Can you work these out from the model? Positions are in its coordinate system, mm. A direction names the side the tool comes from. Give positions to 0.01 mm unless a question says otherwise; leave off trailing zeros. Loops run counter-clockwise (first coordinate to the right, second up) from the corner with the lowest first, then second, coordinate; pieces in that order, holes last. Notation, with made-up numbers: (13, 37.5) - (46, 37.5) arc R17 cw to (46, 41.5) - close; hole circle Ø5 at (49, 89.25). An arc over 180 degrees is marked (long way). Answer as a JSON object with one key per item and string values.
```python
from build123d import *

# Parameters (mm, degrees)
ESBO_O1_W                = 60
ESBO_O1_H                = 50
RESSALTO_EXTRUS_O1_DEPTH = 50
ESBO_O2_W                = 60
ESBO_O2_H                = 29
CORTE_EXTRUS_O1_DEPTH    = 43
FILETE1_R                = 10
FILETE2_R                = 2
ESBO_O3_R                = 1
CORTE_EXTRUS_O2_DEPTH    = 10


with BuildPart() as part:
    # Esboço1 → Ressalto-extrusão1 (new body)
    with BuildSketch(Plane.XY):
        Rectangle(ESBO_O1_W, ESBO_O1_H)
    extrude(amount=RESSALTO_EXTRUS_O1_DEPTH)

    # Esboço2 → Corte-extrusão1 (cut)
    with BuildSketch(Plane.XY.offset(50)):
        Rectangle(ESBO_O2_W, ESBO_O2_H)
    extrude(amount=-CORTE_EXTRUS_O1_DEPTH, mode=Mode.SUBTRACT)

    # Filete1
    filete1_edges = [part.edges().sort_by_distance(p)[0] for p in [
        (0, -14.5, 7),
        (0, 14.5, 7),
    ]]
    fillet(filete1_edges, radius=FILETE1_R)

    # Filete2
    filete2_edges = [part.edges().sort_by_distance(p)[0] for p in [
        (30, -25, 25),
        (-30, -25, 25),
        (-30, 25, 25),
        (30, 25, 25),
    ]]
    fillet(filete2_edges, radius=FILETE2_R)

    # Esboço3 → Corte-extrusão2 (cut)
    with BuildSketch(Plane(origin=(30, 0, 0), x_dir=(0, 0, -1), z_dir=(1, 0, 0))):
        with Locations((-29, -18)):
            Circle(ESBO_O3_R)
        with Locations(Location((-29, 18, 0), (0, 0, 180))):
            Circle(ESBO_O3_R)
    corte_extrus_o2 = extrude(amount=-CORTE_EXTRUS_O2_DEPTH, mode=Mode.SUBTRACT)

    # Espelhar1: Corte-extrusão2 across plane
    add(corte_extrus_o2.mirror(Plane.ZY), mode=Mode.SUBTRACT)


solid = part.part
```
1) If we mould it in two halves opening along Z, with no side actions, what happens to faces 1 (the cylindrical face through (25, 19, 29)), 2 (the flat face through (0, -20, 50)), 3 (the cylindrical face through (29.4, -24.43, 25.35))? For each: released by +Z, released by -Z, zero draft, split by the parting line, or undercut.
Check sheet entries:
{"face 1": "undercut", "face 2": "released by +Z", "face 3": "zero draft"}
2) Imagine slicing it at B-B on x = 6.5. Write out the boundary of the cut face in (y, z), and give its area (3 significant figures).
Check sheet entries:
{"outline": "(-25, 0) - (25, 0) - (25, 50) - (14.5, 50) - (14.5, 17) arc R10 cw to (4.5, 7) - (-4.5, 7) arc R10 cw to (-14.5, 17) - (-14.5, 50) - (-25, 50) - close", "area": "1,300 mm2"}
3) I need wall thicknesses on L1, parallel to Y at x = -27.25, z = 29; L2, parallel to Y at x = 8.5, z = 44.5; L3, parallel to Z at x = 22, y = 18. Which ranges of each line are inside material? Lowest first, please.
Check sheet entries:
{"L1": "-25 to -19, -17 to -14.5, 14.5 to 17, 19 to 25", "L2": "-25 to -14.5, 14.5 to 25", "L3": "0 to 28, 30 to 50"}
4) Imagine slicing it at D-D on z = 29. Write out the boundary of the cut face in (x, y), and give its area (3 significant figures).
Check sheet entries:
{"outline": "(-30, -23) arc R2 ccw to (-28, -25) - (28, -25) arc R2 ccw to (30, -23) - (30, -19) - (20, -19) - (20, -17) - (30, -17) - (30, -14.5) - (-30, -14.5) - (-30, -17) - (-20, -17) - (-20, -19) - (-30, -19) - close; (-30, 14.5) - (30, 14.5) - (30, 17) - (20, 17) - (20, 19) - (30, 19) - (30, 23) arc R2 ccw to (28, 25) - (-28, 25) arc R2 ccw to (-30, 23) - (-30, 19) - (-20, 19) - (-20, 17) - (-30, 17) - close", "area": "1,180 mm2"}
5) Imagine slicing it at A-A on z = 43.5. Write out the boundary of the cut face in (x, y).
Check sheet entries:
{"outline": "(-30, -23) arc R2 ccw to (-28, -25) - (28, -25) arc R2 ccw to (30, -23) - (30, -14.5) - (-30, -14.5) - close; (-30, 14.5) - (30, 14.5) - (30, 23) arc R2 ccw to (28, 25) - (-28, 25) arc R2 ccw to (-30, 23) - close"}
6) Which directions (+Z, -Z, +X, -X, +Y, -Y) give clear straight access to the entire face, cutting with the end or side of a thin tool? Please do faces 4 (the cylindrical face through (-29.43, 24.4, 25.35)), 5 (the flat face through (20, -18, 29)), 6 (the flat face through (0, -14.5, 34)), 7 (the flat face through (-20, -18, 29)).
Check sheet entries:
{"face 4": "+Z, -Z, -X, +Y", "face 5": "+X", "face 6": "+Z, +X, -X", "face 7": "-X"}
7) I'm going to push flat-ended pins straight in: P1, Ø1.6, axis at y = 18, z = 29, coming from the -X side; P2, Ø1.6, axis at y = 18, z = 29, coming from the +X side; P3, Ø8, axis at y = -7.5, z = 31, coming from the +X side (1 decimal); P4, Ø7, axis at x = -5.5, y = -0.5, coming from the +Z side. Where does each tip first touch, or does it pass through?
Check sheet entries:
{"P1": "x = -20", "P2": "x = 20", "P3": "through", "P4": "z = 7"}
8) Imagine slicing it at C-C on y = -1. Write out the boundary of the cut face in (x, z), and give its area (3 significant figures).
Check sheet entries:
{"outline": "(-30, 0) - (30, 0) - (30, 7) - (-30, 7) - close", "area": "420 mm2"}
